Build history of the part. All positions in model axes, mm. Face numbers are marked on the shaded views. A direction names the side the tool comes from. Coordinates: 2 decimals unless noted, no trailing zeros. Order: outer loops, then holes, each group sorted by start corner. A loop starts at its lowest first (then second) coordinate and runs counter-clockwise, first axis right, second up. Notation, with made-up numbers: (-4, 38) -> (51, 38) arc R25 cw to (51, 73) -> close; hole circle Ø3 at (-23.75, 41). An arc over 180 degrees is marked (long way). Write each question's results on one line, items separated by ' | '.
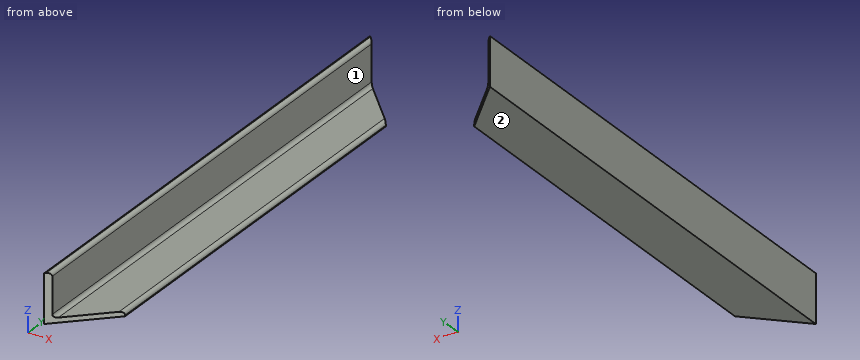
from build123d import *

# Parameters (mm, degrees)
BOSS_EXTRUDE1_DEPTH     = 400
CUT_EXTRUDE1_DEPTH      = 408.622659747
CUT_EXTRUDE1_DEPTH_BACK = 408.622659747


with BuildPart() as part:
    # Sketch1 → Boss-Extrude1 (new body)
    with BuildSketch(Plane(origin=(0, 0, 0), x_dir=(1, 0, 0), z_dir=(0, 1, 0))):
        with BuildLine():
            Line((-27.499872145, 29.213153277), (-67.499872145, 29.213153277))
            Line((-67.499872145, 29.213153277), (-67.499872145, -10.786846723))
            Line((-67.499872145, -10.786846723), (-66.499872145, -10.786846723))
            ThreePointArc((-66.499872145, -10.786846723), (-64.378551801, -9.908167067), (-63.499872145, -7.786846723))
            Line((-63.499872145, -7.786846723), (-63.499872145, 22.213153277))
            ThreePointArc((-63.499872145, 22.213153277), (-62.621192489, 24.334473621), (-60.499872145, 25.213153277))
            Line((-60.499872145, 25.213153277), (-30.499872145, 25.213153277))
            ThreePointArc((-30.499872145, 25.213153277), (-28.378551801, 26.091832933), (-27.499872145, 28.213153277))
            Line((-27.499872145, 28.213153277), (-27.499872145, 29.213153277))
        make_face()
    extrude(amount=BOSS_EXTRUDE1_DEPTH)

    # Sketch2 → Cut-Extrude1 (cut, two sides: drawn at the far end of the back side and taken through both)
    with BuildSketch(Plane(origin=(0, 0, -29.213153277), x_dir=(-1, 0, 0), z_dir=(0, 0, -1)).offset(-CUT_EXTRUDE1_DEPTH_BACK)):
        Polygon((67.499872145, 0), (27.499872145, 40), (27.499872145, 0), align=None)
        Polygon((27.499872145, 400), (67.499872145, 400), (27.499872145, 360), align=None)
    extrude(amount=CUT_EXTRUDE1_DEPTH + CUT_EXTRUDE1_DEPTH_BACK, mode=Mode.SUBTRACT)


solid = part.part
Item 1: Drill centre lines: line 1 (Z direction, x = -55.5, y = 188); line 2 (X direction, y = 62, z = -4.5); line 3 (Y direction, x = -57, z = -27). Where is each one in solid material? Low to high. Write a range as from..to.
Answer:
line 1: z = -29.21..-25.21 | line 2: x = -67.5..-63.5 | line 3: y = 10.5..389.5
Item 2: Pin check, flat tips, straight feed: pin 1 (15 mm diameter, centred on y = 155.5, z = -8.5, fed in from +X); pin 2 (4 mm diameter, centred on x = -37, z = -24, fed in from +Y); pin 3 (5 mm diameter, centred on x = -51, y = 65.5, fed in from +Z). Stop position of each tip, or through.
Answer:
pin 1: stops at x = -63.5 | pin 2: stops at y = 371.09 | pin 3: stops at z = -25.21
Item 3: Slice it at C-C, the plane x = -43. List the corners of the cut face in (y, z), and give its area (3 significant figures).
Answer:
outline: (24.5, -29.21) -> (375.5, -29.21) -> (375.5, -25.21) -> (24.5, -25.21) -> close | area: 1,400 mm^2
Item 4: Slice it at B-B, the plane z = 1.5. List the corners of the cut face in (x, y).
Answer:
outline: (-67.5, 0) -> (-63.5, 4) -> (-63.5, 396) -> (-67.5, 400) -> close
Item 5: Tool access for the marked faces 1 and 2: list every direction of +Z, -Z, +X, -X, +Y, -Y with a clear straight run to the whole face (end or side of a thin tool).
Answer:
face 1: +Z, +X, +Y, -Y | face 2: -Z, +X, -X, +Y, -Y
Item 6: Slice it at A-A, the plane y = 208. List the corners of the cut face in (x, z), and give its area (3 significant figures).
Answer:
outline: (-67.5, -29.21) -> (-27.5, -29.21) -> (-27.5, -28.21) arc R3 ccw to (-30.5, -25.21) -> (-60.5, -25.21) arc R3 cw to (-63.5, -22.21) -> (-63.5, 7.79) arc R3 ccw to (-66.5, 10.79) -> (-67.5, 10.79) -> close | area: 302 mm^2
